Source: CAD feature listing. Evaluate the final solid. Frame: model axes, mm. Round coordinates to 2 decimals unless told otherwise and drop trailing zeros. Write each loop counter-clockwise with the first axis right and the second up, starting at its lowest first coordinate (ties: lowest second). Pieces come first, ordered by that corner, then holes. Notation, with made-up numbers: (-28, 32) - (11, 32) arc R17 cw to (11, 55) - close; hole circle Ø1 at (73, -10). An arc over 180 degrees is marked (long way). Write item = value, one per line. Start each with the question number.
```python
from build123d import *

# Parameters (mm, degrees)
SKETCH1_R           = 2.05
SKETCH1_R_2         = 1.65
BOSS_EXTRUDE1_DEPTH = 3.8


with BuildPart() as part:
    # Sketch1 → Boss-Extrude1 (new body)
    with BuildSketch(Plane.XY):
        with BuildLine():
            Line((0, 3), (-36, 3))
            ThreePointArc((-36, 3), (-39, 0), (-36, -3))
            Line((-36, -3), (0, -3))
            ThreePointArc((0, -3), (3, 0), (0, 3))
        make_face()
        with Locations(Location((0, 0, 0), (0, 0, 180))):
            Circle(SKETCH1_R, mode=Mode.SUBTRACT)
        with Locations(Location((-36, 0, 0), (0, 0, 180))):
            Circle(SKETCH1_R_2, mode=Mode.SUBTRACT)
    extrude(amount=BOSS_EXTRUDE1_DEPTH)


solid = part.part
```
(1) Section A-A (y = 0). Return the cut outline in (x, z), plus the area to 3 significant figures.
(2) Ray query, L1, parallel to Y at x = 0, z = 1.45; L2, parallel to Y at x = -36, z = 1.25; L3, parallel to X at y = 0.6, z = 2.65. Return the intervals inside material, ascending. Write a range as from..to.
(3) Section B-B (z = 1.35). Return the cut outline in (x, y).
(4) Contact query for a flat-ended pin moving along its axis: P1, Ø1.5, axis at y = 1.5, z = 1.5, coming from the +X side. Output: stop coordinate, or through.
(5) Pull-direction query (X, two-part tool) for faces 1 (the cylindrical face through (-34.35, -0.07, 1.87)), 2 (the cylindrical face through (3, 0, 2)), 3 (the flat face through (-18, 0, 3.8)); classes: +X half, -X half, draft (parallel to the pull), parting line (faces both ways), or undercut.
Solution:
q1.outline = (-39, 0) - (-37.65, 0) - (-37.65, 3.8) - (-39, 3.8) - close; (-34.35, 0) - (-2.05, 0) - (-2.05, 3.8) - (-34.35, 3.8) - close; (2.05, 0) - (3, 0) - (3, 3.8) - (2.05, 3.8) - close
q1.area = 131 mm^2
q2.L1 = -3..-2.05, 2.05..3
q2.L2 = -3..-1.65, 1.65..3
q2.L3 = -38.94..-37.54, -34.46..-1.96, 1.96..2.94
q3.outline = (-36, -3) - (0, -3) arc R3 ccw to (0, 3) - (-36, 3) arc R3 ccw to start; hole circle Ø3.3 at (-36, 0); hole circle Ø4.1 at (0, 0)
q4.P1 = 2.9
q5.face_1 = undercut
q5.face_2 = +X half
q5.face_3 = draft
